Job drawing, mm, ordinate dimensions from the low corner. One solid piece. Give positions to 0.01 mm unless a question says otherwise; leave off trailing zeros. Write each loop counter-clockwise with the first axis right and the second up, starting at its lowest first coordinate (ties: lowest second). Pieces come first, ordered by that corner, then holes. Notation, with made-up numbers: M -24.5,81 L 31.5,81 A14 ccw 31.5,86 Z; hole C -32.75,-2.75 d6. An arc over 180 degrees is marked long. Use CSV: the item, a comma, the result in double quotes. Start each with the question number.
Item 1: Drill centre lines: line 1 (X direction, y = 7, z = 0.3); line 2 (Z direction, x = 1.4, y = 7.5) (1 decimal); line 3 (X direction, y = 6.25, z = 0.55). Where is each one in solid material? Low to high. Write a range as [from, to].
Item 2: Cut at C-C (z = 0.6). List the corners of the cut face in (x, y) (1 decimal).
Item 3: Pin check, flat tips, straight feed: pin 1 (1 mm diameter, centred on y = 3, z = 0.5, fed in from -X); pin 2 (1 mm diameter, centred on x = 4, y = 3.5, fed in from -Z); pin 3 (2 mm diameter, centred on x = 2, y = 4, fed in from -Z). Stop position of each tip, or through.
Item 4: Cut at B-B (x = 2.95). List the corners of the cut face in (y, z) (1 decimal), then the cut area to 3 significant figures.
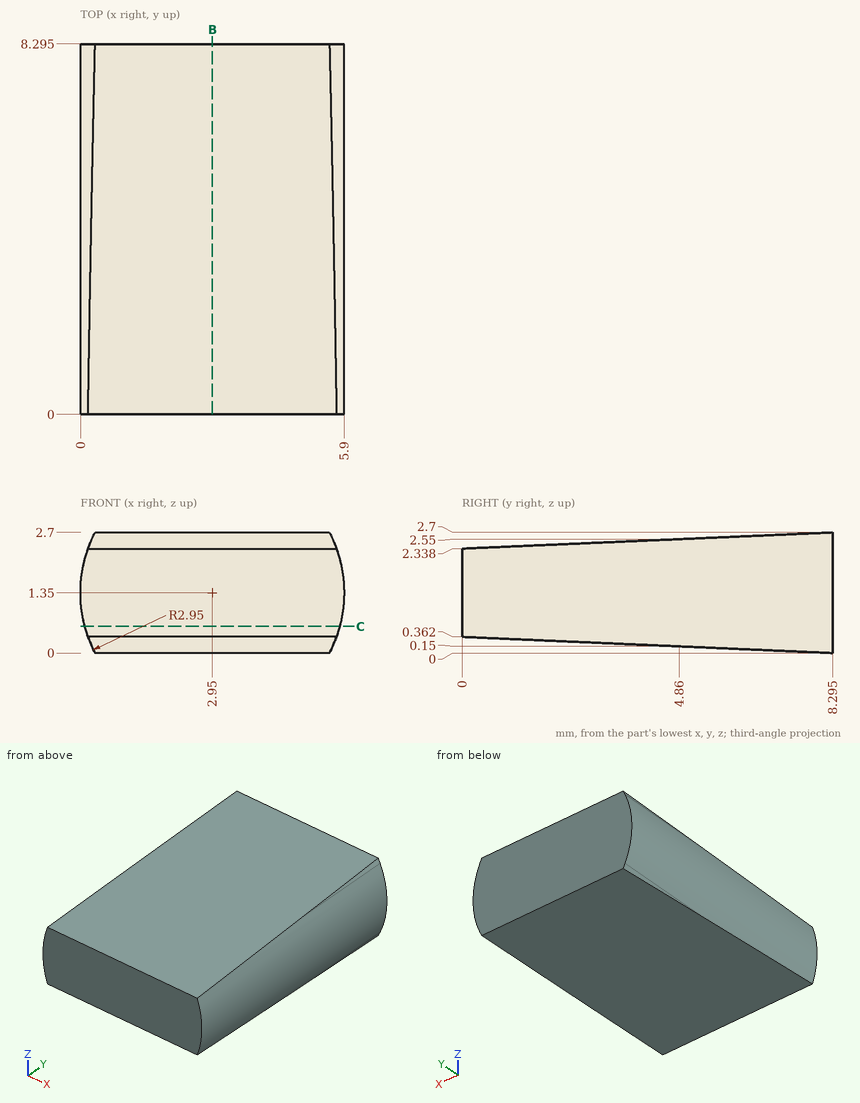
Worked answers:
1,line 1,"x = [0.19, 5.71]"
1,line 2,"z = [0, 2.7]"
1,line 3,"x = [0.11, 5.79]"
2,outline,"M 0.1,0 L 5.8,0 L 5.8,8.3 L 0.1,8.3 Z"
3,pin 1,"stops at x = 0.02"
3,pin 2,"stops at z = 0.19"
3,pin 3,"stops at z = 0.14"
4,outline,"M 0,0.4 L 8.3,0 L 8.3,2.7 L 0,2.3 Z"
4,area,"19.4 mm^2"
